from build123d import *

# Parameters (mm, degrees)
SKETCH1_W           = 135
SKETCH1_H           = 65
BOSS_EXTRUDE1_DEPTH = 37
FILLET1_R           = 2.54
SKETCH2_W           = 11
SKETCH2_H           = 15
BOSS_EXTRUDE2_DEPTH = 23
SKETCH3_W           = 13
SKETCH3_H           = 4
BOSS_EXTRUDE3_DEPTH = 10
SKETCH4_W           = 5
SKETCH4_H           = 5
CUT_EXTRUDE1_DEPTH  = 158.334039546


with BuildPart() as part:
    # Sketch1 → Boss-Extrude1 (new body)
    with BuildSketch(Plane(origin=(0, 0, 0), x_dir=(1, 0, 0), z_dir=(0, 1, 0))):
        with Locations((67.5, -32.5)):
            Rectangle(SKETCH1_W, SKETCH1_H)
    extrude(amount=BOSS_EXTRUDE1_DEPTH)

    # Fillet1
    fillet1_edges = [part.edges().sort_by_distance(p)[0] for p in [
        (135, 37, 32.5),
        (67.5, 37, 0),
        (0, 37, 32.5),
        (67.5, 0, 0),
        (135, 0, 32.5),
        (67.5, 0, 65),
        (0, 0, 32.5),
        (67.5, 37, 65),
        (0, 18.5, 0),
        (135, 18.5, 0),
        (135, 18.5, 65),
        (0, 18.5, 65),
    ]]
    fillet(fillet1_edges, radius=FILLET1_R)

    # Sketch2 → Boss-Extrude2 (add)
    with BuildSketch(Plane(origin=(0, 37, 0), x_dir=(1, 0, 0), z_dir=(0, 1, 0))):
        with Locations((44.5, -11.5)):
            Rectangle(SKETCH2_W, SKETCH2_H)
    extrude(amount=BOSS_EXTRUDE2_DEPTH)

    # Sketch3 → Boss-Extrude3 (add)
    with BuildSketch(Plane(origin=(0, 0, 0), x_dir=(-1, 0, 0), z_dir=(0, 0, -1))):
        with Locations((-59.5, 10)):
            Rectangle(SKETCH3_W, SKETCH3_H)
    extrude(amount=BOSS_EXTRUDE3_DEPTH)

    # Sketch4 → Cut-Extrude1 (cut, through all)
    with BuildSketch(Plane(origin=(0, 12, 0), x_dir=(1, 0, 0), z_dir=(0, 1, 0))):
        with Locations((59.5, 5.5)):
            Rectangle(SKETCH4_W, SKETCH4_H)
    extrude(amount=-CUT_EXTRUDE1_DEPTH, mode=Mode.SUBTRACT)


solid = part.part
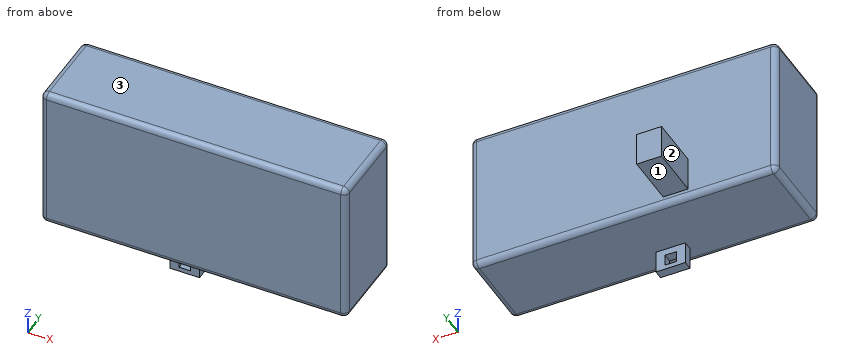
The listing builds one solid part. Answer for the finished solid, in the listing's coordinates (mm). Face numbers are marked on the shaded views. A direction names the side the tool comes from. Coordinates: 2 decimals unless noted, no trailing zeros. Write each loop counter-clockwise with the first axis right and the second up, starting at its lowest first coordinate (ties: lowest second). Pieces come first, ordered by that corner, then holes. Notation, with made-up numbers: (-15.75, -13.5) - (9.25, -13.5) arc R27 cw to (9.25, 9.5) - close; hole circle Ø4 at (88, 1). An arc over 180 degrees is marked (long way). Return JSON: item names as keys, results as strings.
1. The part is cut by section B-B on z = 16. Determine the outline of the cut face in (x, y).
Final values:
{"outline": "(0, 2.54) arc R2.54 ccw to (2.54, 0) - (132.46, 0) arc R2.54 ccw to (135, 2.54) - (135, 34.46) arc R2.54 ccw to (132.46, 37) - (50, 37) - (50, 60) - (39, 60) - (39, 37) - (2.54, 37) arc R2.54 ccw to (0, 34.46) - close"}
2. The part is cut by section A-A on y = 5. Determine the outline of the cut face in (x, z).
Final values:
{"outline": "(0, 2.54) arc R2.54 ccw to (2.54, 0) - (132.46, 0) arc R2.54 ccw to (135, 2.54) - (135, 62.46) arc R2.54 ccw to (132.46, 65) - (2.54, 65) arc R2.54 ccw to (0, 62.46) - close"}
3. Each of these flat-tipped pins is pushed along its axis until it touches: pin 1 Ø12 at (y, z) = (54, 14) entering from -X; pin 2 Ø16.5 at (y, z) = (43, 14) entering from +X; pin 3 Ø12 at (x, y) = (46, 45) entering from -Z. Where does it stop, or does it pass through?
Final values:
{"pin 1": "x = 39", "pin 2": "x = 134.98", "pin 3": "z = 4"}
4. Which of the six approach directions +Z, -Z, +X, -X, +Y, -Y give full straight-line access (tool end or side, diameter ignored) to the marked faces 1, 2 and 3?
Final values:
{"face 1": "-Z, +X, -X, +Y", "face 2": "+Z, -Z, -X, +Y", "face 3": "+Z, +X, -X, +Y, -Y"}
5. Consider line 1 along Y through (x, z) = (6, 59); line 2 along Z through (x, y) = (97.5, 12); line 3 along Z through (x, y) = (62.5, 2). Determine where each line is inside the solid, lowest interval first.
Final values:
{"line 1": "0 to 37", "line 2": "0 to 65", "line 3": "0.06 to 64.94"}
6. The part is cut by section C-C on x = 72. Determine the outline of the cut face in (y, z).
Final values:
{"outline": "(0, 2.54) arc R2.54 ccw to (2.54, 0) - (34.46, 0) arc R2.54 ccw to (37, 2.54) - (37, 62.46) arc R2.54 ccw to (34.46, 65) - (2.54, 65) arc R2.54 ccw to (0, 62.46) - close"}
7. The part is cut by section D-D on y = 49. Determine the outline of the cut face in (x, z), then the cut area to 3 significant figures.
Final values:
{"outline": "(39, 4) - (50, 4) - (50, 19) - (39, 19) - close", "area": "165 mm^2"}
